Check sheet for the modelled part. Datum: model origin and axes. Units: mm. A direction names the side the tool comes from. Coordinates: 2 decimals unless noted, no trailing zeros. Order: outer loops, then holes, each group sorted by start corner. A loop starts at its lowest first (then second) coordinate and runs counter-clockwise, first axis right, second up.
Autodesk Inventor part; units mm, degrees
ref_plane "YZ Plane" through (0, 0, 0) normal (1, 0, 0) x (0, 1, 0)
ref_plane "XZ Plane" through (0, 0, 0) normal (0, 1, 0) x (-1, 0, 0)
ref_plane "XY Plane" through (0, 0, 0) normal (0, 0, 1) x (1, 0, 0)
sketch "Sketch1" plane through (0, 0, 0) normal (0, 1, 0) x (-1, 0, 0)
  line L0 (35, 20) -> (-35, 20)
  line L1 (-35, 20) -> (-35, -20)
  line L2 (-35, -20) -> (35, -20)
  line L3 (35, -20) -> (35, 20)
  line L4 (35, 20) -> (-35, -20) construction
  line L5 (-35, 20) -> (35, -20) construction
  point P0 (0, 0)
  dimension "d0" = 70
  dimension "d1" = 40
extrude "Extrusion1" add sketch "Sketch1" along normal blind 5
sketch "Sketch2" plane through (0, 5, 0) normal (0, 1, 0) x (1, 0, 0)
  circle A0 centre (27.5, -10) radius 2.05
  circle A1 centre (27.5, 10) radius 2.05
  circle A2 centre (-27.5, 10) radius 2.05
  circle A3 centre (-27.5, -10) radius 2.05
  point P0 (0, 0)
  dimension "d4" = 4.1
  dimension "d5" = 27.5
  dimension "d6" = 10
  dimension "d7" = 4.1
  dimension "d8" = 4.1
  dimension "d9" = 4.1
  dimension "d10" = 10
  dimension "d11" = 27.5
  dimension "d12" = 27.5
  dimension "d13" = 10
  dimension "d14" = 10
  dimension "d15" = 27.5
extrude "Extrusion2" cut sketch "Sketch2" against normal blind 5
sketch "Sketch3" plane through (0, 5, 0) normal (0, 1, 0) x (1, 0, 0)
  circle A0 centre (0, 0) radius 12.5
  dimension "d18" = 25
extrude "Extrusion3" cut sketch "Sketch3" against normal blind 5
ref_plane "Work Plane1" through (-35, 0, 0) normal (0, 0, 1) x (1, 0, 0)
sketch "Sketch7" plane through (0, 0, 0) normal (0, -1, 0) x (1, 0, 0)
  line L0 (18, -25) -> (-18, -25)
  line L1 (-18, -25) -> (-18, -20)
  line L2 (-18, -20) -> (18, -20)
  line L3 (18, -20) -> (18, -25)
  line L4 (35, -20) -> (-35, -20)
  point P0 (0, 0)
  dimension "d38" = 36
  dimension "d39" = 5
  dimension "d40" = 18
extrude "Extrusion7" add sketch "Sketch7" against normal blind 45
sketch "Sketch8" plane through (-18, 5, -20) normal (0, 0, 1) x (1, 0, 0)
  line L0 (0, 40) -> (36, 40)
  line L1 (36, 40) -> (36, 20)
  line L2 (36, 20) -> (0, 20)
  line L3 (0, 20) -> (0, 40)
  line L4 (0, 40) -> (36, 40)
  line L5 (0, 0) -> (0, 40)
  line L6 (36, 0) -> (36, 40)
  point P0 (18, -5)
  dimension "d43" = 20
extrude "Extrusion8" add sketch "Sketch8" along normal blind 11
sketch "Sketch9" plane through (35, 0, -20) normal (0, 0, -1) x (-1, 0, 0)
  line L0 (0, 5) -> (17, 5)
  line L1 (17, 5) -> (17, 0)
  line L2 (17, 0) -> (0, 0)
  line L3 (0, 0) -> (0, 5)
  line L4 (53, 5) -> (70, 5)
  line L5 (70, 5) -> (70, 0)
  line L6 (70, 0) -> (53, 0)
  line L7 (53, 0) -> (53, 5)
  line L8 (53, 5) -> (70, 5)
  line L9 (53, 0) -> (53, 45)
  line L10 (53, 0) -> (70, 0)
  line L11 (70, 0) -> (70, 5)
  line L12 (17, 0) -> (17, 45)
  line L13 (0, 5) -> (17, 5)
  line L14 (0, 0) -> (0, 5)
  line L15 (0, 0) -> (17, 0)
  point P0 (35, 0)
extrude "Extrusion9" add sketch "Sketch9" along normal blind 5
sketch "Sketch10" plane through (0, 45, 0) normal (0, 1, 0) x (1, 0, 0)
  circle A0 centre (-10, 20) radius 2.05
  circle A1 centre (10, 20) radius 2.05
  line L0 (18, 25) -> (-18, 25)
  point P0 (0, 0)
  dimension "d48" = 4.1
  dimension "d49" = 4.1
  dimension "d50" = 10
  dimension "d51" = 10
  dimension "d52" = 5
  dimension "d53" = 5
extrude "Extrusion10" cut sketch "Sketch10" against normal blind 10
mirror "Mirror2" about plane through (-35, 0, 0) normal (0, 0, 1) of "Extrusion7", "Extrusion8", "Extrusion9", "Extrusion10"
properties part number "nozzle_bracket" material "ABS Plastic"
(1) Cross-section at D-D (z = -10). Enter the section's corners in (x, y).
Filled in:
outline: (-35, 0) - (-29.55, 0) - (-29.55, 5) - (-35, 5) - close; (-25.45, 0) - (-7.5, 0) - (-7.5, 5) - (-25.45, 5) - close; (-18, 25) - (18, 25) - (18, 45) - (-18, 45) - close; (7.5, 0) - (25.45, 0) - (25.45, 5) - (7.5, 5) - close; (29.55, 0) - (35, 0) - (35, 5) - (29.55, 5) - close
(2) Cross-section at B-B (x = 0). Enter the section's corners in (y, z), and give its area (3 significant figures).
Filled in:
outline: (0, -25) - (45, -25) - (45, -9) - (25, -9) - (25, -20) - (5, -20) - (5, -12.5) - (0, -12.5) - close; (0, 12.5) - (5, 12.5) - (5, 20) - (25, 20) - (25, 9) - (45, 9) - (45, 25) - (0, 25) - close
area: 965 mm2
(3) Cross-section at A-A (y = 14.5). Enter the section's corners in (x, z).
Filled in:
outline: (-18, -25) - (18, -25) - (18, -20) - (-18, -20) - close; (-18, 20) - (18, 20) - (18, 25) - (-18, 25) - close
(4) Go/stop test with flat-tipped pins: P1, Ø17.5, axis at y = 22, z = -20.5, coming from the -X side; P2, Ø6.5, axis at x = -27.5, z = 10, coming from the +Y side; P3, Ø1.2, axis at x = 10, z = -19.5, coming from the +Y side. Record where each tip stops, or that it passes through.
Filled in:
P1: stops at x = -18
P2: stops at y = 5
P3: stops at y = 35
(5) Cross-section at C-C (z = -16.5). Enter the section's corners in (x, y), and give its area (3 significant figures).
Filled in:
outline: (-35, 0) - (35, 0) - (35, 5) - (-35, 5) - close; (-18, 25) - (18, 25) - (18, 45) - (-18, 45) - close
area: 1,070 mm2
(6) Release check for a two-part mould opening along X. For faces 4 (the flat face through (18, 29, 19)), 5 (the cylindrical face through (-29.55, 2.54, 9.91)), 6 (the flat face through (0, 22, 25)) record: +X half, -X half, draft (parallel to the pull), parting line (faces both ways), or undercut.
Filled in:
face 4: +X half
face 5: undercut
face 6: draft
(7) Thickness scan on probe 1 along Z at (x, y) = (10, 37); probe 2 along Z at (x, y) = (-27.5, 1.35); probe 3 along Z at (x, y) = (-11.5, 6.5). Record the ranges inside material, lowest first.
Filled in:
probe 1: z = -25 to -22.05, -17.95 to -9, 9 to 17.95, 22.05 to 25
probe 2: z = -25 to -12.05, -7.95 to 7.95, 12.05 to 25
probe 3: z = -25 to -20, 20 to 25
(8) Tool access check on faces 1 (the flat face through (-18, 29, -19)), 2 (the flat face through (10, 35, 20)), 3 (the flat face through (0, 25, 15)). Record the directions out of +Z, -Z, +X, -X, +Y, -Y that give a thin tool (end or side, any length) a straight path to the whole face; none if there is none.
Filled in:
face 1: +Z, -Z, -X, +Y
face 2: +Y
face 3: +X, -X
